```python
from build123d import *

# Parameters (mm, degrees)
SKETCH_1_R               = 23.4
SKETCH_1_R_2             = 19.8
EXTRUDE_1_DEPTH          = 5
SKETCH_2_W               = 4
SKETCH_2_H               = 2
PATTERN_CIRCULAR_1_COUNT = 23


with BuildPart() as part:
    # 草图1 → 凸台-拉伸1 (new body)
    with BuildSketch(Plane.XY):
        Circle(SKETCH_1_R)
        Circle(SKETCH_1_R_2, mode=Mode.SUBTRACT)
    extrude(amount=EXTRUDE_1_DEPTH)

    # 草图2 → 切除-旋转1 (revolve, cut)
    with BuildSketch(Plane(origin=(21.6, 0, 0), x_dir=(0, 0, -1), z_dir=(1, 0, 0))):
        with Locations((-3.020321316, 1.11760291)):
            Rectangle(SKETCH_2_W, SKETCH_2_H)
    cut_revolve_1 = revolve(axis=Axis((21.6, 0.11760291, 5.020321316), (0, 0, -1)), mode=Mode.SUBTRACT)

    # 阵列(圆周)1: 切除-旋转1 ×23 about axis
    pattern_circular_1_axis = Axis((0, 0, 0), (0, 0, 1))
    for i in range(1, PATTERN_CIRCULAR_1_COUNT):
        add(cut_revolve_1.rotate(pattern_circular_1_axis, i * 360 / PATTERN_CIRCULAR_1_COUNT), mode=Mode.SUBTRACT)


solid = part.part
```
Source: CAD feature listing. Evaluate the final solid. Frame: model axes, mm. A direction names the side the tool comes from. Round coordinates to 2 decimals unless told otherwise and drop trailing zeros. Order: outer loops, then holes, each group sorted by start corner. A loop starts at its lowest first (then second) coordinate and runs counter-clockwise, first axis right, second up. Notation, with made-up numbers: (24, 27.5) -> (45, 27.5) arc R24 ccw to (45, 39.5) -> close; hole circle Ø9 at (29.5, 7.25). An arc over 180 degrees is marked (long way). Use CSV: the item, a comma, the result in double quotes.
(1) Ray query, L1, parallel to X at y = -7, z = 1.5; L2, parallel to X at y = 21, z = 4.3; L3, parallel to Y at x = 0, z = 1.75. Return the intervals inside material, ascending.
Report:
L1,"-22.33 to -20.8, -18.73 to -18.52, 18.52 to 19.3"
L2,"-10.32 to -9.22, -5.47 to -3.52, 0.33 to 2.29, 6.27 to 8.9"
L3,"-23.4 to -23.03, -20.09 to -19.8, 19.8 to 20.33, 22.75 to 23.4"
(2) Section B-B on z = 1.6. Count the separate pieces of the cut face and the enclosed holes in it, and give its area (3 significant figures).
Report:
separate pieces,"23"
enclosed holes,"0"
area,"210 mm^2"
(3) Section A-A on y = 0. Return the cut outline in (x, z), and give its area (3 significant figures).
Report:
outline,"(-23.4, 0) -> (-19.8, 0) -> (-19.8, 5) -> (-23.4, 5) -> close; (19.8, 0) -> (23.4, 0) -> (23.4, 1.02) -> (19.8, 1.02) -> close"
area,"21.7 mm^2"
(4) Access query for faces 1 (the face through (-19, -11, 5)), 2 (the face through (21.517, 2.116, 2.982)). Directions: +Z, -Z, +X, -X, +Y, -Y. A direction counts if a zero-diameter tool reaches every point of the face in a straight line with its end or side. Return the directions, or none.
Report:
face 1,"+Z, +X, -X, +Y, -Y"
face 2,"+Z"
(5) Pull-direction query (Y, two-part tool) for faces 3 (the face through (-3.58, 21.32, 2.98)), 4 (the face through (-20.56, -6.88, 2.98)), 5 (the face through (-15, 16, 5)); classes: +Y half, -Y half, draft (parallel to the pull), parting line (faces both ways), or undercut.
Report:
face 3,"undercut"
face 4,"undercut"
face 5,"draft"
(6) First-contact query: pin 1 Ø1.2 at (x, y) = (10.5, -18.5) entering from +Z; pin 2 Ø3 at (y, z) = (-2.5, 0.5) entering from +X; pin 3 Ø1 at (y, z) = (-11, 2.5) entering from -X. Flat tips, straight axial feed; report the tip coordinate or a pass-through.
Report:
pin 1,"z = 1.02"
pin 2,"x = 23.38"
pin 3,"x = -20.91"
